The model under review builds one solid part; all positions refer to its coordinate system, in mm. A direction names the side the tool comes from. Round coordinates to 2 decimals unless told otherwise and drop trailing zeros. Return JSON: item names as keys, results as strings. Group by question number.
from build123d import *

# Parameters (mm, degrees)
HOLE_WIZARD_2_6_2_6_1_D     = 2.6
HOLE_WIZARD_2_6_2_6_1_DEPTH = 4
HOLE_WIZARD_2_6_2_6_2_D     = 2.6
HOLE_WIZARD_2_6_2_6_2_DEPTH = 6.526692879
HOLE_WIZARD_M80_1_D         = 88.838
HOLE_WIZARD_M80_1_DEPTH     = 27
CHAMFER_1_SIZE              = 0.2


with BuildPart() as part:
    # 草图1 → 旋转1 (revolve)
    with BuildSketch(Plane.XZ):
        with BuildLine():
            Line((47.2599, 27), (0, 27))
            Line((0, 27), (0, 0))
            Line((0, 0), (50.419, 0))
            Line((50.419, 0), (50.419, 5.587))
            Line((50.419, 5.587), (49.04105, 5.587))
            Line((49.04105, 5.587), (50.431651886, 6.547495355))
            ThreePointArc((50.431651886, 6.547495355), (51.1937, 8), (50.431651886, 9.452504645))
            Line((50.431651886, 9.452504645), (49.04105, 10.413))
            Line((49.04105, 10.413), (50.419, 10.413))
            Line((50.419, 10.413), (50.419, 13.587))
            Line((50.419, 13.587), (49.04105, 13.587))
            Line((49.04105, 13.587), (50.431651886, 14.547495355))
            ThreePointArc((50.431651886, 14.547495355), (51.1937, 16), (50.431651886, 17.452504645))
            Line((50.431651886, 17.452504645), (49.04105, 18.413))
            Line((49.04105, 18.413), (50.419, 18.413))
            Line((50.419, 18.413), (50.419, 21))
            Line((50.419, 21), (57.15, 21))
            Line((57.15, 21), (57.15, 27))
            Line((57.15, 27), (50.5587, 27))
            Line((50.5587, 27), (50.5587, 26.279170235))
            Line((50.5587, 26.279170235), (50.013761564, 27.01901462))
            ThreePointArc((50.013761564, 27.01901462), (49.0093, 27.526692879), (48.004838436, 27.01901462))
            Line((48.004838436, 27.01901462), (47.4599, 26.279170235))
            Line((47.4599, 26.279170235), (47.4599, 26.8))
            Line((47.4599, 26.8), (47.2599, 27))
        make_face()
    revolve(axis=Axis((0, 0, 27.526692879), (0, 0, -1)))

    # Ø2.6 (2.6) 直径孔1
    with Locations(Plane(origin=(0, 0, 0), x_dir=(-1, 0, 0), z_dir=(0, 0, -1))):
        with Locations((-33.226947648, 33.226947648), (33.226947648, 33.226947648), (33.226947648, -33.226947648), (-33.226947648, -33.226947648)):
            Hole(HOLE_WIZARD_2_6_2_6_1_D / 2, depth=HOLE_WIZARD_2_6_2_6_1_DEPTH)

    # Ø2.6 (2.6) 直径孔2
    with Locations(Plane(origin=(0, 0, 21), x_dir=(-1, 0, 0), z_dir=(0, 0, -1))):
        with Locations((38.166088515, 38.166088515), (-13.969757959, 52.135846474), (-52.135846474, 13.969757959), (-38.166088515, -38.166088515), (13.969757959, -52.135846474), (52.135846474, -13.969757959)):
            Hole(HOLE_WIZARD_2_6_2_6_2_D / 2, depth=HOLE_WIZARD_2_6_2_6_2_DEPTH)

    # M80 间隙孔1
    with Locations(Plane.XY.offset(27)):
        with Locations((0, 0)):
            Hole(HOLE_WIZARD_M80_1_D / 2, depth=HOLE_WIZARD_M80_1_DEPTH)

    # 倒角1
    chamfer_1_edges = [part.edges().sort_by_distance(p)[0] for p in [
        (-50.419, 0, 0),
        (-50.419, 0, 5.587),
        (-50.419, 0, 10.413),
        (-50.419, 0, 13.587),
        (-50.419, 0, 18.413),
        (-50.5587, 0, 27),
    ]]
    chamfer(chamfer_1_edges, length=CHAMFER_1_SIZE)


solid = part.part
Item 1: Insertion check: pin 1 Ø3.5 at (x, y) = (-38.17, 38.17) entering from -Z; pin 2 Ø3 at (x, y) = (33.23, 33.23) entering from +Z; pin 3 Ø3 at (y, z) = (34.5, 21) entering from +X. Each pin has a flat end and moves straight along its axis. Give the tip position at first contact, or say it passes through.
Item 2: For faces 1 (the face through (-33, -33, 4)), 2 (the face through (-10.9, 48.1, 18.413)), 3 (the face through (-23.879, 37.454, 13.311)), list the 3-axis set-ups (+Z, -Z, +X, -X, +Y, -Y) from which the entire face can be reached by the end or side of a thin tool; tool diameter is ignored.
Item 3: The part is to be moulded in two halves that separate along Y. For faces 4 (the face through (35, 28, 27)), 5 (the face through (-50.37, -2.22, 19.82)), say which applies: +Y half, -Y half, draft (parallel to the pull), parting line (faces both ways), or undercut.
Item 4: Wall thickness on line 1 along Y through (x, z) = (-32.5, 1.5); line 2 along Z through (x, y) = (50.5, -22); line 3 along Y through (x, z) = (7, 11.5): over which ranges is each line inside the solid? List them lowest first.
Values:
{
 "1": {"pin 1": "z = 21", "pin 2": "z = 27.42", "pin 3": "x = 46.66"},
 "2": {"face 1": "-Z", "face 2": "none", "face 3": "+Z, -Z"},
 "3": {"face 4": "undercut", "face 5": "parting line"},
 "4": {"line 1": "-38.55 to -34.3, -32.15 to -30.28, 30.28 to 32.15, 34.3 to 38.55", "line 2": "21 to 27", "line 3": "-49.93 to -43.86, 43.86 to 49.93"}
}
